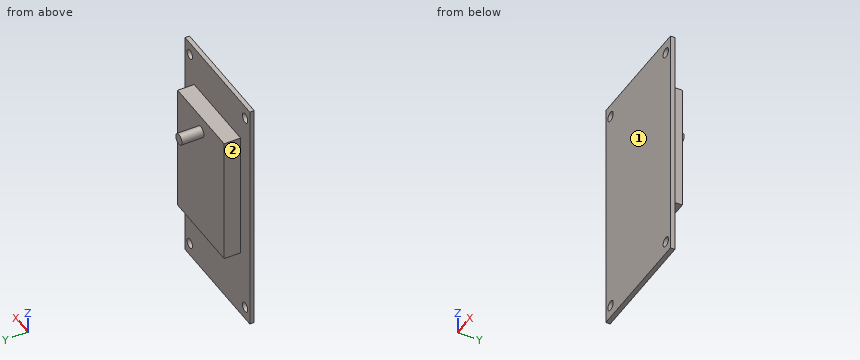
```python
from build123d import *

# Parameters (mm, degrees)
SKETCH1_W           = 42.51
SKETCH1_H           = 87.31
SKETCH1_R           = 1.77
BOSS_EXTRUDE1_DEPTH = 1.6
SKETCH2_W           = 30.51
SKETCH2_H           = 47.31
BOSS_EXTRUDE2_DEPTH = 6
SKETCH4_R           = 2
BOSS_EXTRUDE3_DEPTH = 8


with BuildPart() as part:
    # Sketch1 → Boss-Extrude1 (new body)
    with BuildSketch(Plane(origin=(0, 0, 0), x_dir=(1, 0, 0), z_dir=(0, 1, 0))):
        with Locations((21.255, 43.655)):
            Rectangle(SKETCH1_W, SKETCH1_H)
        with Locations((3.105, 82.605)):
            Circle(SKETCH1_R, mode=Mode.SUBTRACT)
        with Locations((39.405, 82.605)):
            Circle(SKETCH1_R, mode=Mode.SUBTRACT)
        with Locations((3.105, 4.705)):
            Circle(SKETCH1_R, mode=Mode.SUBTRACT)
        with Locations((39.405, 4.705)):
            Circle(SKETCH1_R, mode=Mode.SUBTRACT)
    extrude(amount=BOSS_EXTRUDE1_DEPTH)

    # Sketch2 → Boss-Extrude2 (add)
    with BuildSketch(Plane(origin=(0, 1.6, 0), x_dir=(1, 0, 0), z_dir=(0, 1, 0))):
        with Locations((21.255, 38.655)):
            Rectangle(SKETCH2_W, SKETCH2_H)
    extrude(amount=BOSS_EXTRUDE2_DEPTH)

    # Sketch4 → Boss-Extrude3 (add)
    with BuildSketch(Plane(origin=(0, 7.6, 0), x_dir=(1, 0, 0), z_dir=(0, 1, 0))):
        with Locations((21.255, 21)):
            Circle(SKETCH4_R)
    extrude(amount=BOSS_EXTRUDE3_DEPTH)


solid = part.part
```
Geometry: final body of the model. Coordinates: model frame, mm. Face numbers are marked on the shaded views. A direction names the side the tool comes from. Round coordinates to 2 decimals unless told otherwise and drop trailing zeros. Loops run counter-clockwise (first coordinate to the right, second up) from the corner with the lowest first, then second, coordinate; pieces in that order, holes last.
Item 1: Section C-C, the plane x = 39. Output: boundary loops of the cut face in (y, z), plus the area to 3 significant figures.
Checked values:
outline: (0, -87.31) - (1.6, -87.31) - (1.6, -84.33) - (0, -84.33) - close; (0, -80.88) - (1.6, -80.88) - (1.6, -6.43) - (0, -6.43) - close; (0, -2.98) - (1.6, -2.98) - (1.6, 0) - (0, 0) - close
area: 129 mm2
Item 2: Section A-A, the plane x = 8. Output: boundary loops of the cut face in (y, z), plus the area to 3 significant figures.
Checked values:
outline: (0, -87.31) - (1.6, -87.31) - (1.6, -62.31) - (7.6, -62.31) - (7.6, -15) - (1.6, -15) - (1.6, 0) - (0, 0) - close
area: 424 mm2
Item 3: Section D-D, the plane y = 5.5. Output: boundary loops of the cut face in (x, z), plus the area to 3 significant figures.
Checked values:
outline: (6, -62.31) - (36.51, -62.31) - (36.51, -15) - (6, -15) - close
area: 1,440 mm2
Item 4: Reachability of the marked faces 1 and 2 from +Z, -Z, +X, -X, +Y, -Y: full face, straight path, thin tool, end or side. Return the list, or none.
Checked values:
face 1: +Z, -Z, +X, -X, -Y
face 2: +Z, -Z, -X, +Y
Item 5: Contact query for flat-ended pins moving along their axis: P1, Ø3, axis at x = 22.5, y = 3.5, coming from the -Z side; P2, Ø1.5, axis at y = 5, z = -26, coming from the -X side; P3, Ø4, axis at x = 3.105, z = -4.705, coming from the +Y side. Output: stop coordinate, or through.
Checked values:
P1: stops at z = -62.31
P2: stops at x = 6
P3: stops at y = 1.6
Item 6: Section B-B, the plane z = -21. Output: boundary loops of the cut face in (x, y) (3 decimals).
Checked values:
outline: (0, 0) - (42.51, 0) - (42.51, 1.6) - (36.51, 1.6) - (36.51, 7.6) - (23.255, 7.6) - (23.255, 15.6) - (19.255, 15.6) - (19.255, 7.6) - (6, 7.6) - (6, 1.6) - (0, 1.6) - close
Item 7: Line query: L1, parallel to Y at x = 33, z = -59.5; L2, parallel to X at y = 4, z = -19; L3, parallel to Z at x = 16.5, y = 2.5. Output: solid intervals per line, ascending.
Checked values:
L1: y = 0 to 7.6
L2: x = 6 to 36.51
L3: z = -62.31 to -15
